from build123d import *

# Parameters (mm, degrees)
F1_DEPTH = 38.1
F2_R     = 5.08
F3_T     = -2.54


with BuildPart() as f1:
    # F0 (on Right) → F1 (new body)
    with BuildSketch(Plane.YZ):
        Polygon((12.745309, -23.966217), (27.128007, -0.945347), (14.382698, 23.02087), (-12.745309, 23.966217), (-27.128007, 0.945347), (-14.382698, -23.02087), align=None)
    extrude(amount=-F1_DEPTH)

    # F2
    f2_edges = [f1.edges().sort_by_distance(p)[0] for p in [
        (-19.05, -12.745309, 23.966217),
        (-19.05, -27.128007, 0.945347),
        (-19.05, 14.382698, 23.02087),
        (-19.05, 12.745309, -23.966217),
        (-19.05, 27.128007, -0.945347),
        (-19.05, -14.382698, -23.02087),
        (0, 19.936658, -12.455782),
        (0, 20.755353, 11.037761),
        (0, 0.818695, 23.493543),
        (0, -19.936658, 12.455782),
        (0, -20.755353, -11.037761),
        (0, -0.818695, -23.493543),
    ]]
    fillet(f2_edges, radius=F2_R)

    # F3
    f3_openings = [f1.faces().sort_by_distance(p)[0] for p in [
        (-38.1, 0, 0),
    ]]
    offset(amount=F3_T, openings=f3_openings)


solid = f1.part
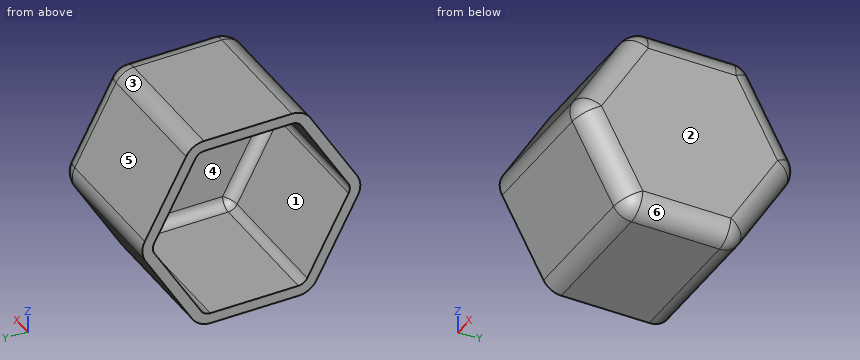
The listing builds one solid part. Answer for the finished solid, in the listing's coordinates (mm). Face numbers are marked on the shaded views. A direction names the side the tool comes from. Coordinates: 2 decimals unless noted, no trailing zeros. Order: outer loops, then holes, each group sorted by start corner. A loop starts at its lowest first (then second) coordinate and runs counter-clockwise, first axis right, second up.
Q1. Given P1, Ø5, axis at x = -34, y = 20, coming from the -Z side; P2, Ø2, axis at y = 5, z = -3.5, coming from the -X side; P3, Ø4, axis at x = -9.5, z = -17, coming from the -Y side, each flat-ended and moving along its own axis, determine where each tip first touches the part or whether it passes through.
Q2. Consider line 1 (X direction, y = -11, z = -2); line 2 (Z direction, x = -28, y = 9.5); line 3 (Y direction, x = -31.5, z = -11.5). Determine where each line is inside the solid, lowest interval first.
Q3. Which of the six approach directions +Z, -Z, +X, -X, +Y, -Y give full straight-line access (tool end or side, diameter ignored) to the marked faces 4, 5 and 6?
Q4. A cutting plane is placed at A-A, the plane x = -28. Write down the section's boundary in (y, z).
Q5. For a pull along Y with two mould halves and no side action, classify the marked faces 1, 2 and 3 as pulls with the +Y half, pulls with the -Y half, needs draft (parallel to the pull), parting line crosses it, or undercut.
Answers follow:
1. P1: stops at z = -16.36
1. P2: stops at x = -2.54
1. P3: stops at y = -18.65
2. line 1: x = -2.54 to 0
2. line 2: z = -23.85 to -21.31, 20.65 to 23.19
2. line 3: y = -20.51 to -17.63, 17.54 to 20.53
3. face 4: -X
3. face 5: +Z, +X, -X, +Y
3. face 6: -Z, +X, -Y
4. outline: (-25.75, -1.64) - (-15.76, -20.43) arc R5.08 ccw to (-11.45, -23.12) - (9.81, -23.86) arc R5.08 ccw to (14.3, -21.48) - (25.57, -3.43) arc R5.08 ccw to (25.75, 1.64) - (15.76, 20.43) arc R5.08 ccw to (11.45, 23.12) - (-9.81, 23.86) arc R5.08 ccw to (-14.3, 21.48) - (-25.57, 3.43) arc R5.08 ccw to start; hole (-23.51, -0.45) - (-13.52, -19.24) arc R2.54 ccw to (-11.36, -20.58) - (9.9, -21.33) arc R2.54 ccw to (12.15, -20.13) - (23.42, -2.09) arc R2.54 ccw to (23.51, 0.45) - (13.52, 19.24) arc R2.54 ccw to (11.36, 20.58) - (-9.9, 21.33) arc R2.54 ccw to (-12.15, 20.13) - (-23.42, 2.09) arc R2.54 ccw to start
5. face 1: undercut
5. face 2: needs draft
5. face 3: pulls with the +Y half
